For this review, take the finished solid that the model builds, in its own axes (mm). Face numbers are marked on the shaded views. A direction names the side the tool comes from. Round coordinates to 2 decimals unless told otherwise and drop trailing zeros. Write each loop counter-clockwise with the first axis right and the second up, starting at its lowest first coordinate (ties: lowest second). Pieces come first, ordered by that corner, then holes. Notation, with made-up numbers: (-32.5, 87.5) - (-7.5, 87.5) arc R18 cw to (-7.5, 121.5) - close; hole circle Ø10 at (53.5, 5). An arc over 180 degrees is marked (long way). One line per item, written item: value. Start each with the question number.
Q1. For probe 1 along Z at (x, y) = (7.75, 2.4); probe 2 along X at (y, z) = (2, 0) (3 decimals); probe 3 along Z at (x, y) = (15.5, 1.55), list the stretches that pass through material, from the lowest coordinate up.
Q2. Tool access review of the marked faces 5, 6 and 7: name each direction out of +Z, -Z, +X, -X, +Y, -Y from which nothing blocks a thin tool from reaching the whole face with its end or side.
Q3. Clearance check with flat-ended pins moving along their axes: pin 1 Ø3.5 at (x, z) = (-25.02, -14.29) entering from +Y; pin 2 Ø3.5 at (x, z) = (24.5, -14) entering from -Y (3 decimals); pin 3 Ø2 at (x, z) = (10.5, -10) entering from +Y (3 decimals); pin 4 Ø19.5 at (x, z) = (0, 0) entering from -Y. State where each tip first meets the part, or that it passes through.
Q4. Add section A-A on y = 7.75. Write out the cut boundary in (x, z).
Q5. Mouldability with a two-part tool opening along X and no side actions: class the marked faces 1, 2, 3 and 4 as +X half, -X half, draft (parallel to the pull), parting line (faces both ways), or undercut.
Q6. Add section D-D on y = 1. Give the number of separate pieces and of enclosed holes in the cut face, and give its area (3 significant figures).
Q7. Add section B-B on x = -7.75. Write out the cut boundary in (y, z) (3 decimals).
Q8. Add section C-C on z = 0. Write out the cut boundary in (x, y) (3 decimals), and give its area (3 significant figures).
```python
from build123d import *

# Parameters (mm, degrees)
SKETCH2_W           = 63.5
SKETCH2_H           = 40.64
SKETCH2_R           = 2.159
SKETCH2_R_2         = 6.125
SKETCH2_R_3         = 1.75
BOSS_EXTRUDE2_DEPTH = 10.16
SKETCH2_4_R         = 2.159
CUT_EXTRUDE1_DEPTH  = 6.985
SKETCH3_R           = 1.75
SKETCH3_R_2         = 6.125
CUT_EXTRUDE2_DEPTH  = 5.715
CHAMFER1_SIZE       = 1.27


with BuildPart() as part:
    # Sketch2 → Boss-Extrude2 (new body)
    with BuildSketch(Plane(origin=(0, 0, 0), x_dir=(1, 0, 0), z_dir=(0, 1, 0))):
        Rectangle(SKETCH2_W, SKETCH2_H)
        with Locations((-25.019, 14.2875)):
            Circle(SKETCH2_R, mode=Mode.SUBTRACT)
        with Locations((25.019, 14.2875)):
            Circle(SKETCH2_R, mode=Mode.SUBTRACT)
        with Locations((25.019, -14.2875)):
            Circle(SKETCH2_R, mode=Mode.SUBTRACT)
        with Locations((-25.019, -14.2875)):
            Circle(SKETCH2_R, mode=Mode.SUBTRACT)
        Circle(SKETCH2_R_2, mode=Mode.SUBTRACT)
        with Locations((7.75, 13.423393759)):
            Circle(SKETCH2_R_3, mode=Mode.SUBTRACT)
        with Locations((15.5, 0)):
            Circle(SKETCH2_R_3, mode=Mode.SUBTRACT)
        with Locations((7.75, -13.423393759)):
            Circle(SKETCH2_R_3, mode=Mode.SUBTRACT)
        with Locations((-7.75, -13.423393759)):
            Circle(SKETCH2_R_3, mode=Mode.SUBTRACT)
        with Locations((-15.5, 0)):
            Circle(SKETCH2_R_3, mode=Mode.SUBTRACT)
        with Locations((-7.75, 13.423393759)):
            Circle(SKETCH2_R_3, mode=Mode.SUBTRACT)
    extrude(amount=BOSS_EXTRUDE2_DEPTH)

    # Sketch2_4 → Cut-Extrude1 (cut)
    with BuildSketch(Plane(origin=(0, 0, 0), x_dir=(1, 0, 0), z_dir=(0, 1, 0))):
        Polygon((-25.019, -10.452681777), (-21.69795, -12.370090889), (-21.69795, -16.204909111), (-25.019, -18.122318223), (-28.34005, -16.204909111), (-28.34005, -12.370090889), align=None)
        with Locations((-25.019, -14.2875)):
            Circle(SKETCH2_4_R, mode=Mode.SUBTRACT)
        Polygon((28.34005, -16.204909111), (28.34005, -12.370090889), (25.019, -10.452681777), (21.69795, -12.370090889), (21.69795, -16.204909111), (25.019, -18.122318223), align=None)
        with Locations((25.019, -14.2875)):
            Circle(SKETCH2_4_R, mode=Mode.SUBTRACT)
        Polygon((25.019, 10.452681777), (21.69795, 12.370090889), (21.69795, 16.204909111), (25.019, 18.122318223), (28.34005, 16.204909111), (28.34005, 12.370090889), align=None)
        with Locations((25.019, 14.2875)):
            Circle(SKETCH2_4_R, mode=Mode.SUBTRACT)
        Polygon((-28.34005, 16.204909111), (-28.34005, 12.370090889), (-25.019, 10.452681777), (-21.69795, 12.370090889), (-21.69795, 16.204909111), (-25.019, 18.122318223), align=None)
        with Locations((-25.019, 14.2875)):
            Circle(SKETCH2_4_R, mode=Mode.SUBTRACT)
    extrude(amount=CUT_EXTRUDE1_DEPTH, mode=Mode.SUBTRACT)

    # Sketch3 → Cut-Extrude2 (cut)
    with BuildSketch(Plane(origin=(0, 10.16, 0), x_dir=(1, 0, 0), z_dir=(0, 1, 0))):
        with BuildLine():
            Line((17.597636205, 20.32), (-17.597636205, 20.32))
            ThreePointArc((-17.597636205, 20.32), (-14.101340421, 18.023940484), (-14.819062067, 13.903157895))
            ThreePointArc((-14.819062067, 13.903157895), (-20.32, 0), (-14.819062067, -13.903157895))
            ThreePointArc((-14.819062067, -13.903157895), (-14.101340421, -18.023940484), (-17.597636205, -20.32))
            Line((-17.597636205, -20.32), (17.597636205, -20.32))
            ThreePointArc((17.597636205, -20.32), (14.101340421, -18.023940484), (14.819062067, -13.903157895))
            ThreePointArc((14.819062067, -13.903157895), (20.32, 0), (14.819062067, 13.903157895))
            ThreePointArc((14.819062067, 13.903157895), (14.101340421, 18.023940484), (17.597636205, 20.32))
        make_face()
        with Locations((-15.5, 0)):
            Circle(SKETCH3_R, mode=Mode.SUBTRACT)
        with Locations((-7.75, -13.423393759)):
            Circle(SKETCH3_R, mode=Mode.SUBTRACT)
        with Locations((7.75, -13.423393759)):
            Circle(SKETCH3_R, mode=Mode.SUBTRACT)
        Circle(SKETCH3_R_2, mode=Mode.SUBTRACT)
        with Locations((15.5, 0)):
            Circle(SKETCH3_R, mode=Mode.SUBTRACT)
        with Locations((-7.75, 13.423393759)):
            Circle(SKETCH3_R, mode=Mode.SUBTRACT)
        with Locations((7.75, 13.423393759)):
            Circle(SKETCH3_R, mode=Mode.SUBTRACT)
        Polygon((-18.310773436, 40.893260665), (-17.597636205, 20.32), (17.597636205, 20.32), (17.597636205, 38.276075745), align=None)
        Polygon((17.597636205, -20.32), (-17.597636205, -20.32), (-25.350098393, -30.312218712), (-13.787636205, -33.380642411), (4.251165531, -33.380642411), (18.013202248, -32.308644201), align=None)
    extrude(amount=-CUT_EXTRUDE2_DEPTH, mode=Mode.SUBTRACT)

    # Chamfer1
    chamfer1_edges = [part.edges().sort_by_distance(p)[0] for p in [
        (24.673818102, 10.16, -20.32),
        (24.673818102, 10.16, 20.32),
        (0, 4.445, -20.32),
        (-20.32, 10.16, 0),
        (-14.101340421, 10.16, 18.023940484),
        (14.101340421, 10.16, -18.023940484),
        (20.32, 10.16, 0),
        (14.101340421, 10.16, 18.023940484),
        (-14.101340421, 10.16, -18.023940484),
        (0, 4.445, 20.32),
        (31.75, 5.08, 20.32),
        (-31.75, 5.08, 20.32),
        (-31.75, 5.08, -20.32),
        (31.75, 5.08, -20.32),
        (31.75, 10.16, 0),
        (-24.673818102, 10.16, -20.32),
        (-31.75, 10.16, 0),
        (-24.673818102, 10.16, 20.32),
    ]]
    chamfer(chamfer1_edges, length=CHAMFER1_SIZE)


solid = part.part
```
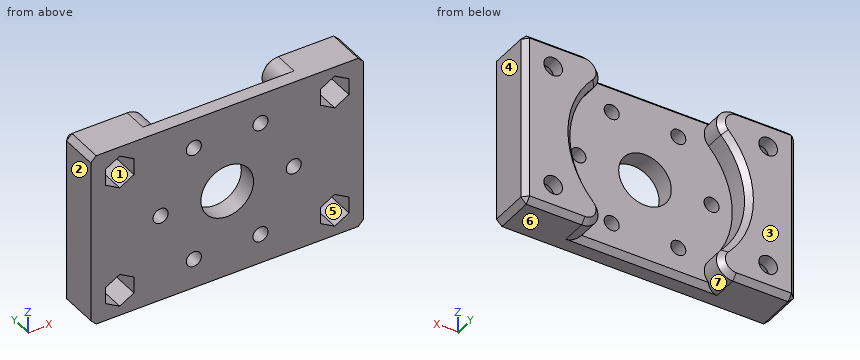
Result set:
1. probe 1: z = -20.32 to -15.17, -11.67 to 11.67, 15.17 to 20.32
1. probe 2: x = -31.75 to -17.25, -13.75 to -6.125, 6.125 to 13.75, 17.25 to 31.75
1. probe 3: z = -20.32 to -1.75, 1.75 to 20.32
2. face 5: -Y
2. face 6: -Z, +X, -X, +Y, -Y
2. face 7: +Y
3. pin 1: passes through
3. pin 2: stops at y = 6.985
3. pin 3: stops at y = 4.445
3. pin 4: stops at y = 0
4. outline: (-31.75, -19.05) - (-30.48, -20.32) - (-17.6, -20.32) arc R3.81 ccw to (-14.82, -13.9) arc R20.32 cw to (-14.82, 13.9) arc R3.81 ccw to (-17.6, 20.32) - (-30.48, 20.32) - (-31.75, 19.05) - close; (14.82, -13.9) arc R3.81 ccw to (17.6, -20.32) - (30.48, -20.32) - (31.75, -19.05) - (31.75, 19.05) - (30.48, 20.32) - (17.6, 20.32) arc R3.81 ccw to (14.82, 13.9) arc R20.32 cw to start; hole circle Ø4.32 at (-25.02, -14.29); hole circle Ø4.32 at (-25.02, 14.29); hole circle Ø4.32 at (25.02, -14.29); hole circle Ø4.32 at (25.02, 14.29)
5. face 1: undercut
5. face 2: -X half
5. face 3: draft
5. face 4: +X half
6. separate pieces: 1
6. enclosed holes: 11
6. area: 2,250 mm^2
7. outline: (0, -20.32) - (3.175, -20.32) - (4.445, -19.05) - (4.445, -15.173) - (0, -15.173) - close; (0, -11.673) - (4.445, -11.673) - (4.445, 11.673) - (0, 11.673) - close; (0, 15.173) - (4.445, 15.173) - (4.445, 19.05) - (3.175, 20.32) - (0, 20.32) - close
8. outline: (-31.75, 0) - (-17.25, 0) - (-17.25, 4.445) - (-20.32, 4.445) - (-20.32, 8.89) - (-21.59, 10.16) - (-30.48, 10.16) - (-31.75, 8.89) - close; (-13.75, 0) - (-6.125, 0) - (-6.125, 4.445) - (-13.75, 4.445) - close; (6.125, 0) - (13.75, 0) - (13.75, 4.445) - (6.125, 4.445) - close; (17.25, 0) - (31.75, 0) - (31.75, 8.89) - (30.48, 10.16) - (21.59, 10.16) - (20.32, 8.89) - (20.32, 4.445) - (17.25, 4.445) - close
8. area: 324 mm^2
